Job drawing, mm, ordinate dimensions from the low corner. One solid piece. Coordinates: 2 decimals unless noted, no trailing zeros. Loops run counter-clockwise (first coordinate to the right, second up) from the corner with the lowest first, then second, coordinate; pieces in that order, holes last. Notation, with made-up numbers: (-1.75, 2) -> (52.25, 2) arc R24 cw to (52.25, 19) -> close; hole circle Ø4 at (59.25, -24). An arc over 180 degrees is marked (long way). Use one line per item in the form item = value. Start each with the question number.
(1) Band-saw the part on B-B on z = 6.35. Count the separate pieces of the cut face and the enclosed holes in it, then the cut area to 3 significant figures.
(2) Band-saw the part on D-D on z = 44.45. Give the cut face in (x, y).
(3) Band-saw the part on A-A on x = 82.55. Give the cut face in (y, z) (3 decimals).
(4) Drill centre lines: L1, parallel to X at y = 1, z = 44.45; L2, parallel to X at y = 1.2, z = 5; L3, parallel to Z at x = 82.55, y = 0.6 (3 decimals). Where is each one in solid material? Low to high. Write a range as [from, to].
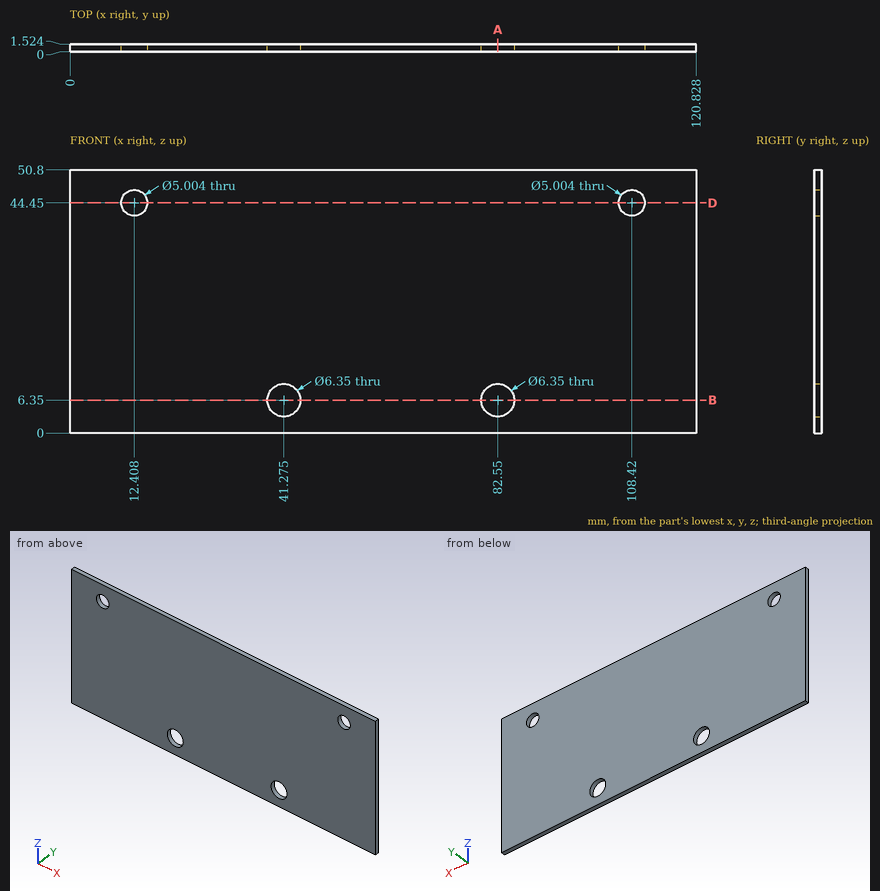
A:
q1.separate_pieces = 3
q1.enclosed_holes = 0
q1.area = 165 mm²
q2.outline = (0, 0) -> (9.91, 0) -> (9.91, 1.52) -> (0, 1.52) -> close; (14.91, 0) -> (105.92, 0) -> (105.92, 1.52) -> (14.91, 1.52) -> close; (110.92, 0) -> (120.83, 0) -> (120.83, 1.52) -> (110.92, 1.52) -> close
q3.outline = (0, 0) -> (1.524, 0) -> (1.524, 3.175) -> (0, 3.175) -> close; (0, 9.525) -> (1.524, 9.525) -> (1.524, 50.8) -> (0, 50.8) -> close
q4.L1 = [0, 9.91], [14.91, 105.92], [110.92, 120.83]
q4.L2 = [0, 38.4], [44.15, 79.68], [85.42, 120.83]
q4.L3 = [0, 3.175], [9.525, 50.8]
